Here's the drawing with two shaded views (mm, measured from the low corner). I have some questions. Coordinates: 2 decimals unless noted, no trailing zeros. Write each loop counter-clockwise with the first axis right and the second up, starting at its lowest first coordinate (ties: lowest second). Pieces come first, ordered by that corner, then holes. Notation, with made-up numbers: (86.25, 55) -> (110.25, 55) arc R25 cw to (110.25, 93) -> close; hole circle Ø4 at (49, 5). An arc over 180 degrees is marked (long way). Put each result on its own line as item: value.
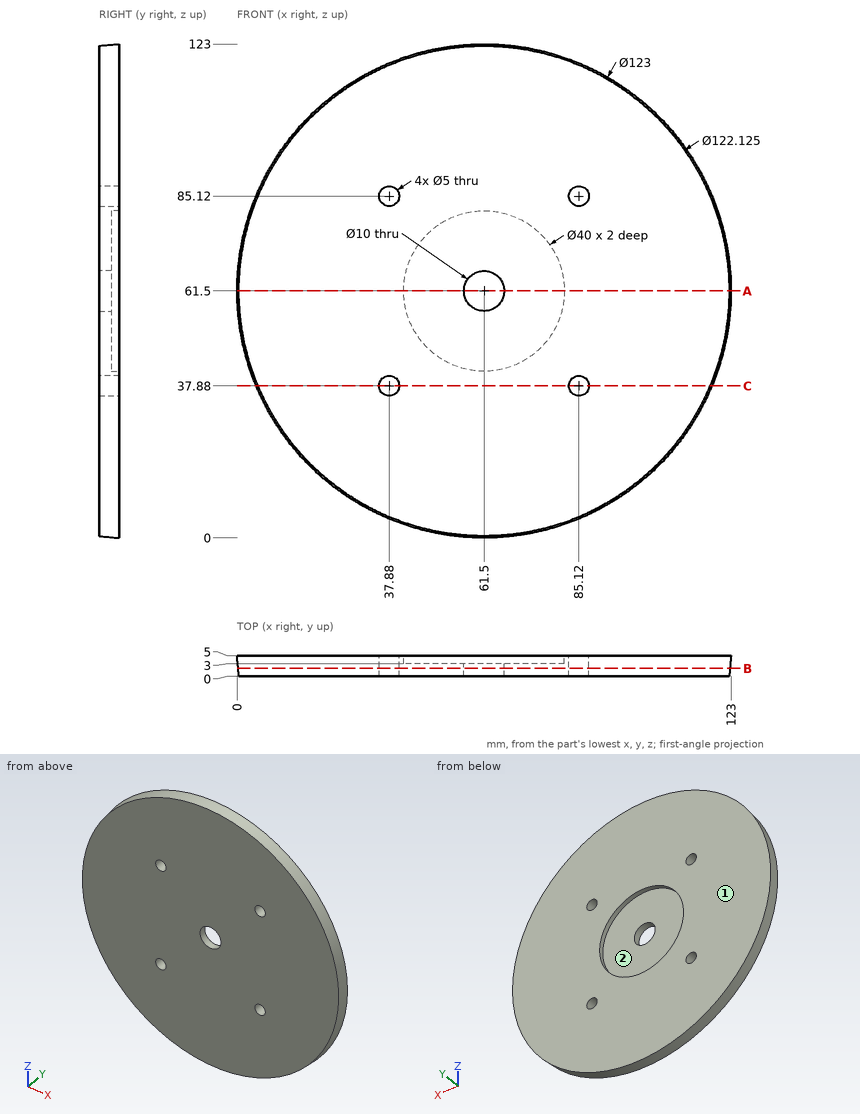
Item 1: For P1, Ø2, axis at y = 3, z = 29, coming from the +X side (1 decimal); P2, Ø12, axis at x = 70, z = 62.5, coming from the +Y side, each with a flat end and sliding along its axis, tell me the tip position at first contact or that it passes through.
Output:
P1: stops at x = 114.1
P2: stops at y = 3
Item 2: Please list where these lines run through material, in increasing order: line 1 along X through (y, z) = (1.7, 37.88); line 2 along Z through (x, y) = (37.88, 3.6); line 3 along X through (y, z) = (1.35, 85.12). Write a range as from..to.
Output:
line 1: x = 5.03..35.38, 40.38..82.62, 87.62..117.97
line 2: z = 4.85..35.38, 40.38..82.62, 87.62..118.15
line 3: x = 5.06..35.38, 40.38..82.62, 87.62..117.94
Item 3: If we mould it in two halves opening along Z, with no side actions, what happens to the marked faces 1 and 2? For each: released by +Z, released by -Z, zero draft, split by the parting line, or undercut.
Output:
face 1: zero draft
face 2: undercut
Item 4: Imagine slicing it at C-C on z = 37.88. State how many separate pieces and enclosed holes the cut face has.
Output:
separate pieces: 3
enclosed holes: 0
Item 5: Imagine slicing it at B-B on y = 1.9. Write out the boundary of the cut face in (x, z).
Output:
outline: circle Ø122.46 at (61.5, 61.5); hole circle Ø5 at (37.88, 37.88); hole circle Ø5 at (37.88, 85.12); hole circle Ø10 at (61.5, 61.5); hole circle Ø5 at (85.12, 37.88); hole circle Ø5 at (85.12, 85.12)
Item 6: Imagine slicing it at A-A on z = 61.5. Write out the boundary of the cut face in (x, y), then the cut area to 3 significant figures.
Output:
outline: (0, 5) -> (0.44, 0) -> (56.5, 0) -> (56.5, 3) -> (41.5, 3) -> (41.5, 5) -> close; (66.5, 0) -> (122.56, 0) -> (123, 5) -> (81.5, 5) -> (81.5, 3) -> (66.5, 3) -> close
area: 503 mm²
